```python
from build123d import *

# Parameters (mm, degrees)
F0_W     = 40
F0_H     = 40
F1_DEPTH = 80
F2_W     = 10
F2_H     = 64
F3_DEPTH = 15
F6_R     = 2.85
F7_DEPTH = 8


with BuildPart() as f1:
    # F0 (on Top) → F1 (new body)
    with BuildSketch(Plane.XY):
        Rectangle(F0_W, F0_H)
    extrude(amount=F1_DEPTH)


with BuildPart() as f3:
    # F2 (on face) → F3 (new body)
    with BuildSketch(Plane.YZ.offset(20)):
        with Locations((-10, 40)):
            Rectangle(F2_W, F2_H)
        with Locations((10, 40)):
            Rectangle(F2_W, F2_H)
    extrude(amount=-F3_DEPTH)


with BuildPart() as f4_1:
    # F4: instance of F3
    add(f3.part.mirror(Plane.YZ))


with BuildPart() as f1_1:
    add(f1.part)

    # F5: cut F3, F4_1
    add(f3.part, mode=Mode.SUBTRACT)
    add(f4_1.part, mode=Mode.SUBTRACT)


with BuildPart() as f7:
    # F6 (on face) → F7 (new body, through all)
    with BuildSketch(Plane.XY.offset(80)):
        with Locations((12.5, -10)):
            Circle(F6_R)
        with Locations((12.5, 10)):
            Circle(F6_R)
        with Locations((-12.5, 10)):
            Circle(F6_R)
        with Locations((-12.5, -10)):
            Circle(F6_R)
    extrude(amount=-F7_DEPTH)


with BuildPart() as f9_1:
    # F9: instance of F7
    add(f7.part.mirror(Plane(origin=(12.5, 10, 40), x_dir=(1, 0, 0), z_dir=(0, 0, 1))))


with BuildPart() as f1_2:
    add(f1_1.part)

    # F10: cut F7, F9_1
    add(f7.part, mode=Mode.SUBTRACT)
    add(f9_1.part, mode=Mode.SUBTRACT)


solid = f1_2.part
```
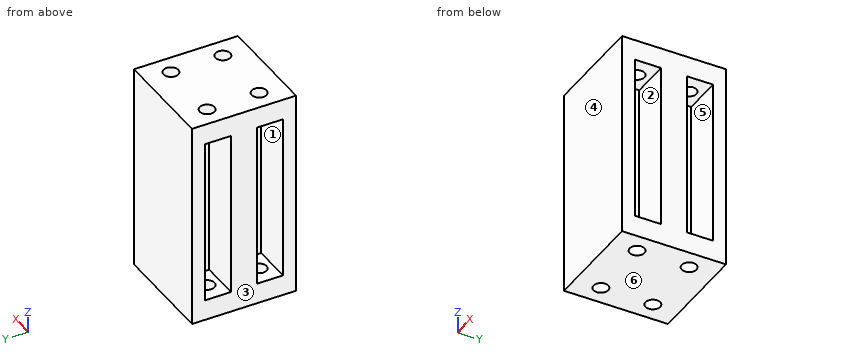
Geometry: final body of the model. Coordinates: model frame, mm. Face numbers are marked on the shaded views. A direction names the side the tool comes from. Round coordinates to 2 decimals unless told otherwise and drop trailing zeros. Loops run counter-clockwise (first coordinate to the right, second up) from the corner with the lowest first, then second, coordinate; pieces in that order, holes last.
Item 1: Line query: L1, parallel to Y at x = 12, z = 35; L2, parallel to Y at x = 12.5, z = 2.25; L3, parallel to X at y = -11, z = 76. Output: solid intervals per line, ascending.
Checked values:
L1: y = -20 to -15, -5 to 5, 15 to 20
L2: y = -20 to -12.85, -7.15 to 7.15, 12.85 to 20
L3: x = -20 to -15.17, -9.83 to 9.83, 15.17 to 20
Item 2: Contact query for flat-ended pins moving along their axis: P1, Ø8, axis at y = -10, z = 48, coming from the -X side; P2, Ø3, axis at y = 9, z = 50.5, coming from the +X side. Output: stop coordinate, or through.
Checked values:
P1: stops at x = -5
P2: stops at x = 5
Item 3: Section A-A, the plane x = -12.5. Output: boundary loops of the cut face in (y, z), plus the area to 3 significant figures.
Checked values:
outline: (-20, 0) - (-12.85, 0) - (-12.85, 8) - (-15, 8) - (-15, 72) - (-12.85, 72) - (-12.85, 80) - (-20, 80) - close; (-7.15, 0) - (7.15, 0) - (7.15, 8) - (5, 8) - (5, 72) - (7.15, 72) - (7.15, 80) - (-7.15, 80) - (-7.15, 72) - (-5, 72) - (-5, 8) - (-7.15, 8) - close; (12.85, 0) - (20, 0) - (20, 80) - (12.85, 80) - (12.85, 72) - (15, 72) - (15, 8) - (12.85, 8) - close
area: 1,740 mm2
Item 4: Section B-B, the plane y = -10. Output: boundary loops of the cut face in (x, z).
Checked values:
outline: (-20, 0) - (-15.35, 0) - (-15.35, 8) - (-20, 8) - close; (-20, 72) - (-15.35, 72) - (-15.35, 80) - (-20, 80) - close; (-9.65, 0) - (9.65, 0) - (9.65, 8) - (5, 8) - (5, 72) - (9.65, 72) - (9.65, 80) - (-9.65, 80) - (-9.65, 72) - (-5, 72) - (-5, 8) - (-9.65, 8) - close; (15.35, 0) - (20, 0) - (20, 8) - (15.35, 8) - close; (15.35, 72) - (20, 72) - (20, 80) - (15.35, 80) - close
Item 5: Mould query, pull axis Y, two halves, no side actions, for the marked faces 4, 5 and 6. Classes: released by +Y, released by -Y, zero draft, split by the parting line, or undercut.
Checked values:
face 4: released by -Y
face 5: undercut
face 6: zero draft
Item 6: Reachability of the marked faces 1, 2 and 3 from +Z, -Z, +X, -X, +Y, -Y: full face, straight path, thin tool, end or side. Return the list, or none.
Checked values:
face 1: -X
face 2: +X
face 3: +Z, -Z, -X, +Y, -Y
Item 7: Section C-C, the plane x = 7.5. Output: boundary loops of the cut face in (y, z).
Checked values:
outline: (-20, 0) - (20, 0) - (20, 80) - (-20, 80) - close; hole (-15, 8) - (-5, 8) - (-5, 72) - (-15, 72) - close; hole (5, 8) - (15, 8) - (15, 72) - (5, 72) - close
Item 8: Section D-D, the plane z = 39. Output: boundary loops of the cut face in (x, y).
Checked values:
outline: (-20, -20) - (20, -20) - (20, -15) - (5, -15) - (5, -5) - (20, -5) - (20, 5) - (5, 5) - (5, 15) - (20, 15) - (20, 20) - (-20, 20) - (-20, 15) - (-5, 15) - (-5, 5) - (-20, 5) - (-20, -5) - (-5, -5) - (-5, -15) - (-20, -15) - close
